Work out the finished part from the listing and answer in its coordinate system (mm). Face numbers are marked on the shaded views. A direction names the side the tool comes from. Give positions to 0.01 mm unless a question says otherwise; leave off trailing zeros. Loops run counter-clockwise (first coordinate to the right, second up) from the corner with the lowest first, then second, coordinate; pieces in that order, holes last. Notation, with made-up numbers: (-29.5, 7.5) - (24.5, 7.5) arc R21 cw to (24.5, 39.5) - close; hole circle Ø4 at (85, 31.25). An arc over 180 degrees is marked (long way). Use one line per item in the form item = value. Start each with the question number.
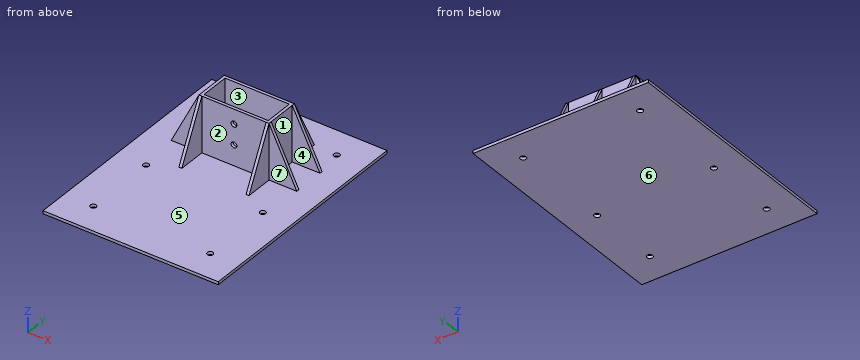
from build123d import *

# Parameters (mm, degrees)
F0_W         = 5
F0_H         = 50
F0_H_2       = 5
F0_W_2       = 50
F0_W_3       = 110
F1_DEPTH     = 100
F0_W_4       = 300
F0_H_3       = 400
F2_DEPTH     = 5
F3_T4_DEPTH  = 522.9657747574
F3_T9_DEPTH  = 522.9657747574
F3_T14_DEPTH = 522.9657747574
F3_T19_DEPTH = 522.9657747574
F3_T24_DEPTH = 522.9657747574
F3_T29_DEPTH = 522.9657747574
F3_T34_DEPTH = 522.9657747574
F3_T39_DEPTH = 522.9657747574
F3_T44_DEPTH = 522.9657747574
F6_D         = 10
F6_DEPTH     = 20
F6_TIP       = 3.0043030951
F7_D         = 10
F7_DEPTH     = 20
F7_TIP       = 3.0043030951


# Not quite as in the source:
# - a fillet or chamfer that OpenCascade refuses, or shapes differently, is made with other operations: its cross-section is extruded or revolved along the edge and cut away or added


with BuildPart() as f1:
    # F0 (on Top) → F1 (new body)
    with BuildSketch(Plane.XY):
        with Locations((-57.5, 130)):
            Rectangle(F0_W, F0_H)
        with Locations((-57.5, 20)):
            Rectangle(F0_W, F0_H)
        with Locations((-57.5, 102.5)):
            Rectangle(F0_W, F0_H_2)
        with Locations((57.5, 102.5)):
            Rectangle(F0_W, F0_H_2)
        with Locations((-85, 47.5)):
            Rectangle(F0_W_2, F0_H_2)
        with Locations((-85, 102.5)):
            Rectangle(F0_W_2, F0_H_2)
        Polygon((-55, 105), (-55, 100), (55, 100), (55, 105), (2.5, 105), (-2.5, 105), align=None)
        with Locations((57.5, 47.5)):
            Rectangle(F0_W, F0_H_2)
        with Locations((57.5, 75)):
            Rectangle(F0_W, F0_H)
        with Locations((0, 47.5)):
            Rectangle(F0_W_3, F0_H_2)
        with Locations((57.5, 130)):
            Rectangle(F0_W, F0_H)
        with Locations((85, 102.5)):
            Rectangle(F0_W_2, F0_H_2)
        with Locations((-57.5, 47.5)):
            Rectangle(F0_W, F0_H_2)
        with Locations((85, 47.5)):
            Rectangle(F0_W_2, F0_H_2)
        with Locations((-57.5, 75)):
            Rectangle(F0_W, F0_H)
        with Locations((57.5, 20)):
            Rectangle(F0_W, F0_H)
        with Locations((0, 130)):
            Rectangle(F0_W, F0_H)
    extrude(amount=F1_DEPTH)

    # F0 (on Top) → F2 (join)
    with BuildSketch(Plane.XY):
        Rectangle(F0_W_4, F0_H_3)
        Polygon((55, 45), (-55, 45), (-55, -5), (-60, -5), (-60, 45), (-110, 45), (-110, 50), (-60, 50), (-60, 100), (-110, 100), (-110, 105), (-60, 105), (-60, 155), (-55, 155), (-55, 105), (-2.5, 105), (-2.5, 155), (2.5, 155), (2.5, 105), (55, 105), (55, 155), (60, 155), (60, 105), (110, 105), (110, 100), (60, 100), (60, 50), (110, 50), (110, 45), (60, 45), (60, -5), (55, -5), align=None, mode=Mode.SUBTRACT)
        with Locations((0, 75)):
            Rectangle(F0_W_3, F0_H)
    extrude(amount=F2_DEPTH)

    # F3: chamfer of 50 x 100 on 9 edges, made by hand


with BuildPart() as f3_tool2:
    # F3_s3 → F3_t4 (new body)
    with BuildSketch(Plane.XZ.offset(213.9828873787)):
        Polygon((60, 100), (110, 0), (110, 100), align=None)
    extrude(amount=-F3_T4_DEPTH)

    split(bisect_by=Plane.XY.offset(5), keep=Keep.TOP)


with BuildPart() as f1_1:
    add(f1.part)

    # F3_t1: cut F3_tool2
    add(f3_tool2.part, mode=Mode.SUBTRACT)


with BuildPart() as f3_tool7:
    # F3_s8 → F3_t9 (new body)
    with BuildSketch(Plane.XZ.offset(158.9828873787)):
        Polygon((60, 100), (110, 0), (110, 100), align=None)
    extrude(amount=-F3_T9_DEPTH)

    split(bisect_by=Plane.XY.offset(5), keep=Keep.TOP)


with BuildPart() as f1_2:
    add(f1_1.part)

    # F3_t6: cut F3_tool7
    add(f3_tool7.part, mode=Mode.SUBTRACT)


with BuildPart() as f3_tool12:
    # F3_s13 → F3_t14 (new body)
    with BuildSketch(Plane.YZ.offset(-203.9828873787)):
        Polygon((45, 100), (-5, 0), (-5, 100), align=None)
    extrude(amount=F3_T14_DEPTH)

    split(bisect_by=Plane.XY.offset(5), keep=Keep.TOP)


with BuildPart() as f1_3:
    add(f1_2.part)

    # F3_t11: cut F3_tool12
    add(f3_tool12.part, mode=Mode.SUBTRACT)


with BuildPart() as f3_tool17:
    # F3_s18 → F3_t19 (new body)
    with BuildSketch(Plane.YZ.offset(318.9828873787)):
        Polygon((105, 100), (155, 0), (155, 100), align=None)
    extrude(amount=-F3_T19_DEPTH)

    split(bisect_by=Plane.XY.offset(5), keep=Keep.TOP)


with BuildPart() as f1_4:
    add(f1_3.part)

    # F3_t16: cut F3_tool17
    add(f3_tool17.part, mode=Mode.SUBTRACT)


with BuildPart() as f3_tool22:
    # F3_s23 → F3_t24 (new body)
    with BuildSketch(Plane.YZ.offset(-318.9828873787)):
        Polygon((45, 100), (-5, 0), (-5, 100), align=None)
    extrude(amount=F3_T24_DEPTH)

    split(bisect_by=Plane.XY.offset(5), keep=Keep.TOP)


with BuildPart() as f1_5:
    add(f1_4.part)

    # F3_t21: cut F3_tool22
    add(f3_tool22.part, mode=Mode.SUBTRACT)


with BuildPart() as f3_tool27:
    # F3_s28 → F3_t29 (new body)
    with BuildSketch(Plane.XZ.offset(-308.9828873787)):
        Polygon((-60, 100), (-110, 0), (-110, 100), align=None)
    extrude(amount=F3_T29_DEPTH)

    split(bisect_by=Plane.XY.offset(5), keep=Keep.TOP)


with BuildPart() as f1_6:
    add(f1_5.part)

    # F3_t26: cut F3_tool27
    add(f3_tool27.part, mode=Mode.SUBTRACT)


with BuildPart() as f3_tool32:
    # F3_s33 → F3_t34 (new body)
    with BuildSketch(Plane.XZ.offset(-363.9828873787)):
        Polygon((-60, 100), (-110, 0), (-110, 100), align=None)
    extrude(amount=F3_T34_DEPTH)

    split(bisect_by=Plane.XY.offset(5), keep=Keep.TOP)


with BuildPart() as f1_7:
    add(f1_6.part)

    # F3_t31: cut F3_tool32
    add(f3_tool32.part, mode=Mode.SUBTRACT)


with BuildPart() as f3_tool37:
    # F3_s38 → F3_t39 (new body)
    with BuildSketch(Plane.YZ.offset(203.9828873787)):
        Polygon((155, 0), (105, 100), (155, 100), align=None)
    extrude(amount=-F3_T39_DEPTH)

    split(bisect_by=Plane.XY.offset(5), keep=Keep.TOP)


with BuildPart() as f1_8:
    add(f1_7.part)

    # F3_t36: cut F3_tool37
    add(f3_tool37.part, mode=Mode.SUBTRACT)


with BuildPart() as f3_tool42:
    # F3_s43 → F3_t44 (new body)
    with BuildSketch(Plane.YZ.offset(261.4828873787)):
        Polygon((105, 100), (155, 0), (155, 100), align=None)
    extrude(amount=-F3_T44_DEPTH)

    split(bisect_by=Plane.XY.offset(5), keep=Keep.TOP)


with BuildPart() as f1_9:
    add(f1_8.part)

    # F3_t41: cut F3_tool42
    add(f3_tool42.part, mode=Mode.SUBTRACT)

    # F6
    with Locations(Plane.XZ.offset(-44.9998)):
        with Locations((0, 40), (0, 75)):
            Hole(F6_D / 2, depth=F6_DEPTH)
            with Locations((0, 0, -(F6_DEPTH + F6_TIP / 2))):  # 118° drill point
                Cone(0, F6_D / 2, F6_TIP, mode=Mode.SUBTRACT)

    # F7
    with Locations(Plane(origin=(0, 0, 0), x_dir=(1, 0, 0), z_dir=(0, 0, -1))):
        with Locations((-100, 25), (-100, -150), (100, -150), (100, 25), (100, 150), (-100, 150)):
            Hole(F7_D / 2, depth=F7_DEPTH)
            with Locations((0, 0, -(F7_DEPTH + F7_TIP / 2))):  # 118° drill point
                Cone(0, F7_D / 2, F7_TIP, mode=Mode.SUBTRACT)


solid = f1_9.part
1) A cutting plane is placed at B-B (y = -150). Give the vertices of the cut face in (x, z), plus the area to 3 significant figures.
2) A cutting plane is placed at C-C (y = 19). Give the vertices of the cut face in (x, z).
3) A cutting plane is placed at D-D (x = -47). Give the vertices of the cut face in (y, z).
4) Determine the mould class of the marked faces 1, 2, 3 and 4 for opening direction X: released by +X, released by -X, zero draft, split by the parting line, or undercut.
5) A cutting plane is placed at A-A (x = -100). Give the vertices of the cut face in (y, z), plus the area to 3 significant figures.
6) Flat-ended cylindrical pins translate along their axes: pin 1 Ø10 at (y, z) = (71.5, 62.5) entering from -X; pin 2 Ø14.5 at (x, z) = (-85, 45) entering from +Y; pin 3 Ø3 at (x, z) = (31.5, 89.5) entering from -Y. Find the tip coordinate at first contact, or state that the pin passes through.
7) A tool of negligible diameter and unlimited length cuts with its end or side. For the marked faces 5, 6 and 7, from which of +Z, -Z, +X, -X, +Y, -Y can it reach the whole face along a straight path? Write none if from no direction.
8) Find the intervals of material crossed by probe 1 along Z at (x, y) = (0, 48.85); probe 2 along Y at (x, z) = (-100, 3.9); probe 3 along X at (y, z) = (-150, 2.55), in increasing order.
Answer sheet:
q1.outline = (-150, 0) - (-105, 0) - (-105, 5) - (-150, 5) - close; (-95, 0) - (95, 0) - (95, 5) - (-95, 5) - close; (105, 0) - (150, 0) - (150, 5) - (105, 5) - close
q1.area = 1,400 mm²
q2.outline = (-150, 0) - (150, 0) - (150, 5) - (60, 5) - (60, 48) - (55, 48) - (55, 5) - (-55, 5) - (-55, 48) - (-60, 48) - (-60, 5) - (-150, 5) - close
q3.outline = (-200, 0) - (200, 0) - (200, 5) - (105, 5) - (105, 100) - (100, 100) - (100, 5) - (50, 5) - (50, 100) - (45, 100) - (45, 5) - (-200, 5) - close
q4.face_1 = released by +X
q4.face_2 = undercut
q4.face_3 = undercut
q4.face_4 = zero draft
q5.outline = (-200, 0) - (-155, 0) - (-155, 5) - (-200, 5) - close; (-145, 0) - (-30, 0) - (-30, 5) - (-145, 5) - close; (-20, 0) - (145, 0) - (145, 5) - (105, 5) - (105, 20) - (100, 20) - (100, 5) - (50, 5) - (50, 20) - (45, 20) - (45, 5) - (-20, 5) - close; (155, 0) - (200, 0) - (200, 5) - (155, 5) - close
q5.area = 2,000 mm²
q6.pin_1 = -60
q6.pin_2 = 105
q6.pin_3 = 45
q7.face_5 = +Z
q7.face_6 = -Z, +X, -X, +Y, -Y
q7.face_7 = +Z, +X, -Y
q8.probe_1 = 0 to 35, 45 to 70, 80 to 100
q8.probe_2 = -200 to -155, -145 to -30, -20 to 145, 155 to 200
q8.probe_3 = -150 to -105, -95 to 95, 105 to 150
